The figure shows three views and two pictorial views of one solid part (mm, origin at its lowest corner). Answer the questions. A direction names the side the tool comes from. Coordinates: 2 decimals unless noted, no trailing zeros. Order: outer loops, then holes, each group sorted by start corner. A loop starts at its lowest first (then second) coordinate and runs counter-clockwise, first axis right, second up. Notation, with made-up numbers: (-21.5, 62.5) -> (0.5, 62.5) arc R19 ccw to (0.5, 94.5) -> close; hole circle Ø2 at (39.5, 2). An arc over 180 degrees is marked (long way). Write item = value, one per line. Start each with the question number.
Q1. For a pull along X with two mould halves and no side action, classify the marked faces 1, 2, 3 and 4 as +X half, -X half, draft (parallel to the pull), parting line (faces both ways), or undercut.
Q2. The part is cut by section D-D, the plane x = 6. Determine the outline of the cut face in (y, z).
Q3. Which of the six approach directions +Z, -Z, +X, -X, +Y, -Y give full straight-line access (tool end or side, diameter ignored) to the marked faces 5 and 6?
Q4. Flat-ended cylindrical pins translate along their axes: pin 1 (1 mm diameter, centred on x = 8.5, y = 8, fed in from +Z); pin 2 (10 mm diameter, centred on x = 20, y = 4.5, fed in from -Z); pin 3 (6 mm diameter, centred on x = 8, y = 4, fed in from -Z); pin 4 (2.5 mm diameter, centred on x = 33.5, y = 12.5, fed in from -Z). Find the tip coordinate at first contact, or state that the pin passes through.
Q5. The part is cut by section B-B, the plane z = 12.5. Determine the outline of the cut face in (x, y), plus the area to 3 significant figures.
Q6. Straight lines are drawn through the part: L1, parallel to X at y = 12.5, z = 15.5; L2, parallel to X at y = 21, z = 18; L3, parallel to Y at x = 33.5, z = 9.75. For each, find the intervals that lie inside material, in ascending order. Write a range as from..to.
Q7. The part is cut by section C-C, the plane x = 33.5. Determine the outline of the cut face in (y, z).
Q8. The part is cut by section A-A, the plane y = 12.5. Determine the outline of the cut face in (x, z).
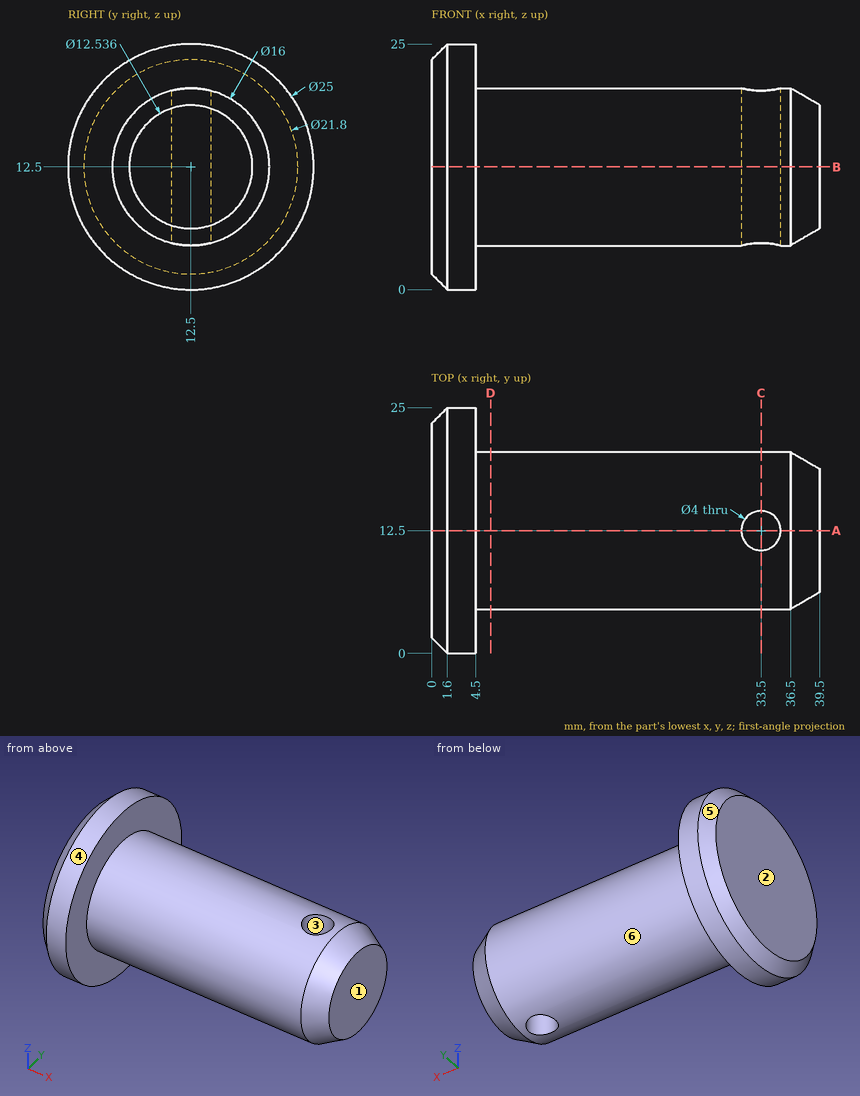
Model answer:
q1.face_1 = +X half
q1.face_2 = -X half
q1.face_3 = undercut
q1.face_4 = draft
q2.outline = circle Ø16 at (12.5, 12.5)
q3.face_5 = -X
q3.face_6 = +X
q4.pin_1 = 19.43
q4.pin_2 = 5.08
q4.pin_3 = 6.69
q4.pin_4 = through
q5.outline = (0, 1.6) -> (1.6, 0) -> (4.5, 0) -> (4.5, 4.5) -> (36.5, 4.5) -> (39.5, 6.23) -> (39.5, 18.77) -> (36.5, 20.5) -> (4.5, 20.5) -> (4.5, 25) -> (1.6, 25) -> (0, 23.4) -> close; hole circle Ø4 at (33.5, 12.5)
q5.area = 652 mm2
q6.L1 = 0..31.5, 35.5..39.5
q6.L2 = 0..4.5
q6.L3 = 4.99..10.5, 14.5..20.01
q7.outline = (10.5, 4.75) -> (10.5, 20.25) arc R8 ccw to start; (14.5, 4.75) arc R8 ccw to (14.5, 20.25) -> close
q8.outline = (0, 1.6) -> (1.6, 0) -> (4.5, 0) -> (4.5, 4.5) -> (31.5, 4.5) -> (31.5, 20.5) -> (4.5, 20.5) -> (4.5, 25) -> (1.6, 25) -> (0, 23.4) -> close; (35.5, 4.5) -> (36.5, 4.5) -> (39.5, 6.23) -> (39.5, 18.77) -> (36.5, 20.5) -> (35.5, 20.5) -> close
